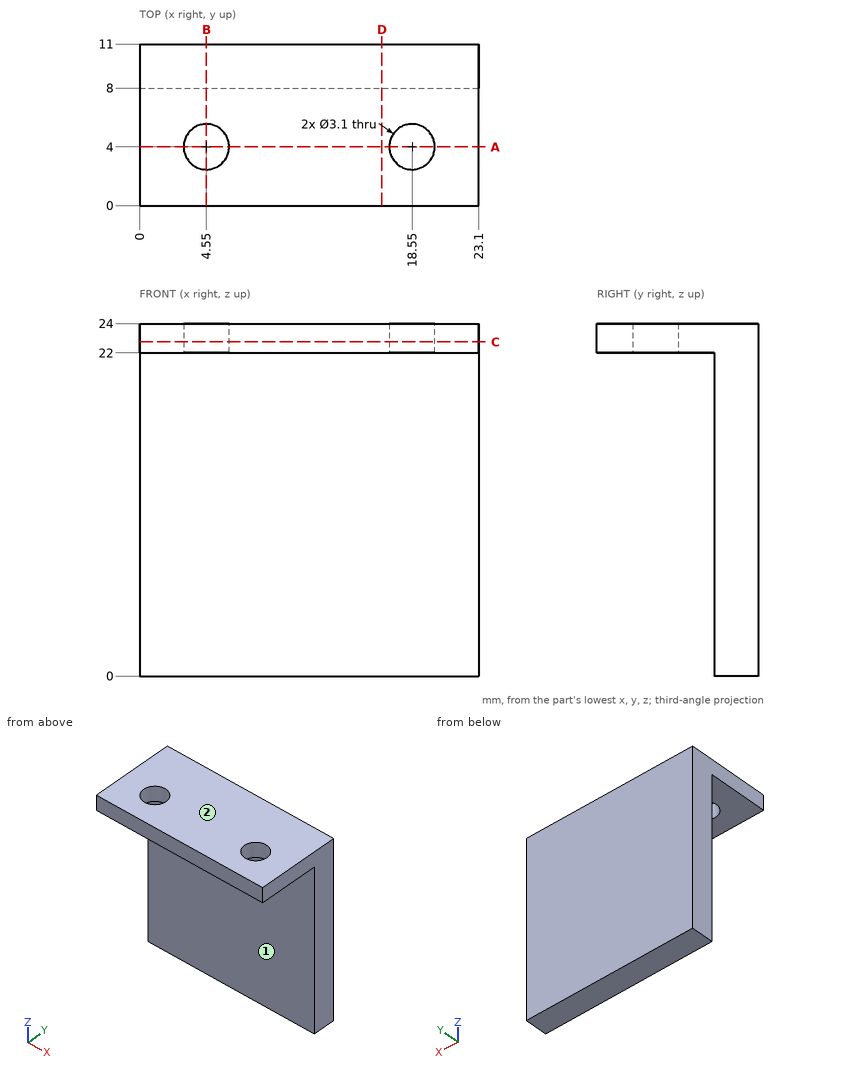
Here's the drawing with two shaded views (mm, measured from the low corner). I have some questions. A direction names the side the tool comes from. Round coordinates to 2 decimals unless told otherwise and drop trailing zeros. Loops run counter-clockwise (first coordinate to the right, second up) from the corner with the lowest first, then second, coordinate; pieces in that order, holes last. Notation, with made-up numbers: (70.25, 72.25) - (78.25, 72.25) arc R23 ccw to (78.25, 84.25) - close; hole circle Ø1 at (38, -35.5). An arc over 180 degrees is marked (long way). Use CSV: the item, a comma, the result in double quotes.
Item 1: If we section it at A-A on y = 4: List the corners of the cut face in (x, z) for me, then the cut area to 3 significant figures.
Here are the results:
outline,"(0, 22) - (3, 22) - (3, 24) - (0, 24) - close; (6.1, 22) - (17, 22) - (17, 24) - (6.1, 24) - close; (20.1, 22) - (23.1, 22) - (23.1, 24) - (20.1, 24) - close"
area,"33.8 mm²"
Item 2: If we section it at B-B on x = 4.55: List the corners of the cut face in (y, z) for me.
Here are the results:
outline,"(0, 22) - (2.45, 22) - (2.45, 24) - (0, 24) - close; (5.55, 22) - (8, 22) - (8, 0) - (11, 0) - (11, 24) - (5.55, 24) - close"
Item 3: For the marked faces 1 and 2, which set-ups out of +Z, -Z, +X, -X, +Y, -Y let a thin tool reach every point of the face, with its end or its side?
Here are the results:
face 1,"-Z, +X, -X, -Y"
face 2,"+Z, +X, -X, +Y, -Y"
Item 4: If we section it at D-D on x = 16.5: List the corners of the cut face in (y, z) for me, then the cut area to 3 significant figures.
Here are the results:
outline,"(0, 22) - (8, 22) - (8, 0) - (11, 0) - (11, 24) - (0, 24) - close"
area,"88.0 mm²"
Item 5: Will these pins go through, and if not, where does the flat tip stop? pin 1 (3 mm diameter, centred on x = 18.55, y = 4, fed in from +Z); pin 2 (2.5 mm diameter, centred on x = 6, y = 6, fed in from -Z); pin 3 (1.5 mm diameter, centred on x = 20.5, z = 21, fed in from -Y); pin 4 (3 mm diameter, centred on y = 9.5, z = 14, fed in from -X).
Here are the results:
pin 1,"passes through"
pin 2,"stops at z = 22"
pin 3,"stops at y = 8"
pin 4,"stops at x = 0"
Item 6: I need wall thicknesses on L1, parallel to Y at x = 18.55, z = 22.5; L2, parallel to Y at x = 5.75, z = 15.25; L3, parallel to Z at x = 3.25, y = 1. Which ranges of each line are inside material? Lowest first, please. Write a range as [from, to].
Here are the results:
L1,"y = [0, 2.45], [5.55, 11]"
L2,"y = [8, 11]"
L3,"z = [22, 24]"
Item 7: If we section it at C-C on z = 22.75: List the corners of the cut face in (x, y) for me, then the cut area to 3 significant figures.
Here are the results:
outline,"(0, 0) - (23.1, 0) - (23.1, 11) - (0, 11) - close; hole circle Ø3.1 at (4.55, 4); hole circle Ø3.1 at (18.55, 4)"
area,"239 mm²"
